```python
from build123d import *

# Parameters (mm, degrees)
SKETCH1_W           = 230
SKETCH1_H           = 30
BOSS_EXTRUDE1_DEPTH = 10
SKETCH2_R           = 1
CUT_EXTRUDE1_DEPTH  = 54
SKETCH3_W           = 25
SKETCH3_H           = 10
BOSS_EXTRUDE2_DEPTH = 54
FILLET1_R           = 10
SKETCH4_W           = 60
SKETCH4_H           = 30
BOSS_EXTRUDE3_DEPTH = 15
CUT_EXTRUDE3_DEPTH  = 40
BOSS_EXTRUDE4_DEPTH = 30
FILLET2_R           = 5
FILLET3_R           = 10


with BuildPart() as part:
    # Sketch1 → Boss-Extrude1 (new body)
    with BuildSketch(Plane.XY):
        Rectangle(SKETCH1_W, SKETCH1_H)
    extrude(amount=BOSS_EXTRUDE1_DEPTH)

    # Sketch2 → Cut-Extrude1 (cut)
    with BuildSketch(Plane(origin=(0, 15, 0), x_dir=(1, 0, 0), z_dir=(0, 1, 0))):
        with Locations(Location((50, -5, 0), (0, 0, 180))):
            Circle(SKETCH2_R)
        with Locations(Location((100, -5, 0), (0, 0, 180))):
            Circle(SKETCH2_R)
        with Locations(Location((-100, -5, 0), (0, 0, 180))):
            Circle(SKETCH2_R)
        with Locations(Location((-50, -5, 0), (0, 0, 180))):
            Circle(SKETCH2_R)
    extrude(amount=-CUT_EXTRUDE1_DEPTH, mode=Mode.SUBTRACT)

    # Sketch3 → Boss-Extrude2 (add)
    with BuildSketch(Plane.XZ.offset(15)):
        with Locations((-75, 5)):
            Rectangle(SKETCH3_W, SKETCH3_H)
    extrude(amount=BOSS_EXTRUDE2_DEPTH)

    # Fillet1
    fillet1_edges = [part.edges().sort_by_distance(p)[0] for p in [
        (-87.5, -15, 5),
        (-62.5, -15, 5),
    ]]
    fillet(fillet1_edges, radius=FILLET1_R)

    # Sketch4 → Boss-Extrude3 (add, symmetric)
    with BuildSketch(Plane.XZ.offset(69)):
        with Locations((-75, 15)):
            Rectangle(SKETCH4_W, SKETCH4_H)
    extrude(amount=BOSS_EXTRUDE3_DEPTH, both=True)

    # Sketch6 → Cut-Extrude3 (cut)
    with BuildSketch(Plane.XZ.offset(84)):
        Polygon((-105, 30), (-105, 14.999997289), (-90, 30), align=None)
        Polygon((-90, 0), (-105, 14.999997289), (-105, 0), align=None)
        Polygon((-45, 30), (-60, 30), (-45, 14.999997289), align=None)
        Polygon((-45, 14.999997289), (-60, 0), (-45, 0), align=None)
    extrude(amount=-CUT_EXTRUDE3_DEPTH, mode=Mode.SUBTRACT)

    # Sketch7 → Boss-Extrude4 (add)
    with BuildSketch(Plane.XZ.offset(84)):
        Polygon((-75, 30), (-90, 45.499997289), (-90, 30), align=None)
        Polygon((-60, 45.499997289), (-75, 30), (-60, 30), align=None)
    extrude(amount=-BOSS_EXTRUDE4_DEPTH)

    # Fillet2
    fillet2_edges = [part.edges().sort_by_distance(p)[0] for p in [
        (-45, -69, 14.999997289),
        (-60, -69, 30),
        (-105, -69, 14.999997289),
        (-90, -69, 30),
    ]]
    fillet(fillet2_edges, radius=FILLET2_R)

    # Fillet3
    fillet3_edges = [part.edges().sort_by_distance(p)[0] for p in [
        (-62.5, -54, 5),
        (-87.5, -54, 5),
        (-75, -54, 10),
    ]]
    fillet(fillet3_edges, radius=FILLET3_R)


solid = part.part
```
The listing builds one solid part. Answer for the finished solid, in the listing's coordinates (mm). A direction names the side the tool comes from. Round coordinates to 2 decimals unless told otherwise and drop trailing zeros. Loops run counter-clockwise (first coordinate to the right, second up) from the corner with the lowest first, then second, coordinate; pieces in that order, holes last.
Q1. Section B-B, the plane z = 37.5 is taken. Determine the outline of the cut face in (x, y).
Q2. Find the intervals of material crossed by line 1 (Z direction, x = 100, y = -1); line 2 (Z direction, x = -54.5, y = 9); line 3 (X direction, y = -62.5, z = 40), in increasing order.
Q3. Given pin 1 Ø1.8 at (x, z) = (50, 5) entering from -Y; pin 2 Ø3 at (y, z) = (-30.5, 3) entering from -X; pin 3 Ø12 at (x, z) = (-36, 13) entering from -Y; pin 4 Ø10.5 at (y, z) = (-71, 36.5) entering from -X, each flat-ended and moving along its own axis, determine where each tip first touches the part or whether it passes through.
Q4. Section C-C, the plane x = -85 is taken. Determine the outline of the cut face in (y, z), then the cut area to 3 significant figures.
Q5. For a pull along X with two mould halves and no side action, classify faces 6 (the face through (-47.07, -68.79, 15.05)), 7 (the face through (-87.5, -34, 5)), 8 (the face through (-67.395, -69.21, 37.858)) as released by +X, released by -X, zero draft, split by the parting line, or undercut.
Q6. Which of the six approach directions +Z, -Z, +X, -X, +Y, -Y give full straight-line access (tool end or side, diameter ignored) to faces 1 (the face through (-90.51, -51.15, 7.92)), 2 (the face through (-96, -68, 6)), 3 (the face through (-90, -69, 39)), 4 (the face through (115, 0, 5)), 5 (the face through (-59.49, -51.15, 7.92))?
Q7. Section A-A, the plane y = 8.5 is taken. Determine the outline of the cut face in (x, z).
Q8. Section D-D, the plane z = 16 is taken. Determine the outline of the cut face in (x, y).
Completed:
1. outline: (-90, -84) - (-82.26, -84) - (-82.26, -54) - (-90, -54) - close; (-67.74, -84) - (-60, -84) - (-60, -54) - (-67.74, -54) - close
2. line 1: z = 0 to 4, 6 to 10
2. line 2: z = 0 to 10
2. line 3: x = -90 to -84.68, -65.32 to -60
3. pin 1: passes through
3. pin 2: stops at x = -87.5
3. pin 3: stops at y = -15
3. pin 4: stops at x = -90.07
4. outline: (-84, 0) - (15, 0) - (15, 10) - (-44, 10) arc R10 cw to (-54, 20) - (-54, 40.33) - (-84, 40.33) - close
4. area: 1,920 mm2
5. face 6: released by +X
5. face 7: released by -X
5. face 8: undercut
6. face 1: +Z, -Z, -X
6. face 2: -Z, -X, -Y
6. face 3: +Z, -X, +Y, -Y
6. face 4: +Z, -Z, +X, +Y, -Y
6. face 5: +Z, -Z, +X
7. outline: (-115, 0) - (115, 0) - (115, 10) - (-115, 10) - close; hole circle Ø2 at (-100, 5); hole circle Ø2 at (-50, 5); hole circle Ø2 at (50, 5); hole circle Ø2 at (100, 5)
8. outline: (-102.83, -84) - (-47.17, -84) - (-47.17, -54) - (-52.5, -54) arc R10 cw to (-56.5, -53.17) - (-93.5, -53.17) arc R10 cw to (-97.5, -54) - (-102.83, -54) - close
